```python
from build123d import *

# Parameters (mm, degrees)
BOSS_EXTRUDE1_DEPTH            = 2
F_3_1_3_1_DIAMETER_HOLE1_D     = 3.1
F_3_1_3_1_DIAMETER_HOLE1_DEPTH = 10
F_3_1_3_1_DIAMETER_HOLE1_TIP   = 0.931333959


with BuildPart() as part:
    # Sketch1 → Boss-Extrude1 (new body)
    with BuildSketch(Plane(origin=(0, 0, 0), x_dir=(1, 0, 0), z_dir=(0, 1, 0))):
        Polygon((0, 0), (0, 40), (7.5, 40), (7.5, 15), (28.5, 15), (28.5, 0), align=None)
    extrude(amount=BOSS_EXTRUDE1_DEPTH)

    # Ø3.1 (3.1) Diameter Hole1
    with Locations(Plane(origin=(0, 2, 0), x_dir=(1, 0, 0), z_dir=(0, 1, 0))):
        with Locations((10.5, 5), (25.5, 5)):
            Hole(F_3_1_3_1_DIAMETER_HOLE1_D / 2, depth=F_3_1_3_1_DIAMETER_HOLE1_DEPTH)
            with Locations((0, 0, -(F_3_1_3_1_DIAMETER_HOLE1_DEPTH + F_3_1_3_1_DIAMETER_HOLE1_TIP / 2))):  # 118° drill point
                Cone(0, F_3_1_3_1_DIAMETER_HOLE1_D / 2, F_3_1_3_1_DIAMETER_HOLE1_TIP, mode=Mode.SUBTRACT)


solid = part.part
```
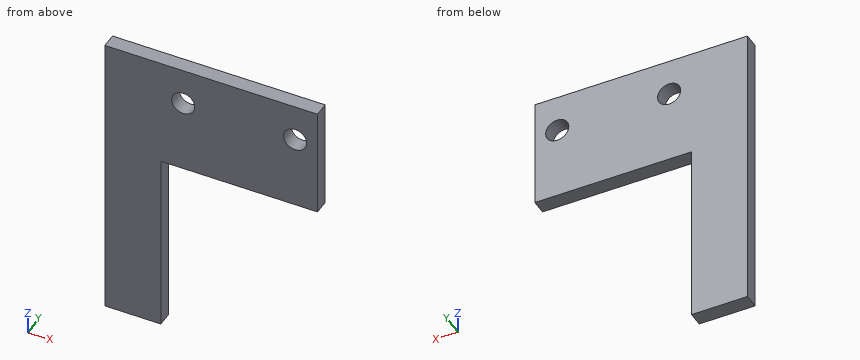
Can you work these out from the model? Positions are in its coordinate system, mm. Give positions to 0.01 mm unless a question says otherwise; leave off trailing zeros. Order: outer loops, then holes, each group sorted by start corner. A loop starts at its lowest first (then second) coordinate and runs counter-clockwise, first axis right, second up. Notation, with made-up numbers: (23, -3.75) - (49, -3.75) arc R23 cw to (49, 29.25) - close; hole circle Ø3 at (-3, 82). An arc over 180 degrees is marked (long way). Use a Markdown table: item, result. Add a question column.
Q1. If we section it at C-C on y = 1.5: Write out the boundary of the cut face in (x, z), plus the area to 3 significant figures.
Q2. I'm going to push flat-ended pins straight in: pin 1 (1 mm diameter, centred on x = 13.5, y = 0.5, fed in from -Z); pin 2 (8 mm diameter, centred on x = 13, z = -16.5, fed in from +Y); pin 3 (1 mm diameter, centred on y = 1, z = -24, fed in from +X). Where does each tip first touch, or does it pass through?
Q3. If we section it at D-D on z = -27: Write out the boundary of the cut face in (x, y).
Q4. If we section it at B-B on z = -5: Write out the boundary of the cut face in (x, y).
Q5. Please list where these lines run through material, in increasing order: line 1 along X through (y, z) = (1, -5); line 2 along Z through (x, y) = (25.5, 0.7); line 3 along Z through (x, y) = (14, 0.45).
Q6. If we section it at A-A on x = 25.5: Write out the boundary of the cut face in (y, z).
Answers follow:
| question | item | result |
|---|---|---|
| 1 | outline | (0, -40) - (7.5, -40) - (7.5, -15) - (28.5, -15) - (28.5, 0) - (0, 0) - close; hole circle Ø3.1 at (10.5, -5); hole circle Ø3.1 at (25.5, -5) |
| 1 | area | 600 mm^2 |
| 2 | pin 1 | stops at z = -15 |
| 2 | pin 2 | stops at y = 2 |
| 2 | pin 3 | stops at x = 7.5 |
| 3 | outline | (0, 0) - (7.5, 0) - (7.5, 2) - (0, 2) - close |
| 4 | outline | (0, 0) - (8.95, 0) - (8.95, 2) - (0, 2) - close; (12.05, 0) - (23.95, 0) - (23.95, 2) - (12.05, 2) - close; (27.05, 0) - (28.5, 0) - (28.5, 2) - (27.05, 2) - close |
| 5 | line 1 | x = 0 to 8.95, 12.05 to 23.95, 27.05 to 28.5 |
| 5 | line 2 | z = -15 to -6.55, -3.45 to 0 |
| 5 | line 3 | z = -15 to 0 |
| 6 | outline | (0, -15) - (2, -15) - (2, -6.55) - (0, -6.55) - close; (0, -3.45) - (2, -3.45) - (2, 0) - (0, 0) - close |
